The drawing under review shows one solid part. Ordinate dimensions are in mm from its lowest x, y, z. A direction names the side the tool comes from. Coordinates: 2 decimals unless noted, no trailing zeros. Write each loop counter-clockwise with the first axis right and the second up, starting at its lowest first coordinate (ties: lowest second). Pieces come first, ordered by that corner, then holes. Notation, with made-up numbers: (72, 13.25) - (93, 13.25) arc R20 ccw to (93, 50.25) - close; hole circle Ø2 at (61, -17.5). An arc over 180 degrees is marked (long way). Put each result on its own line as item: value. Start each with the question number.
Item 1: Consider section C-C on x = 86. Give the boundary of the cut face in (y, z), then the cut area to 3 significant figures.
Item 2: Consider section B-B on y = 80. Give the boundary of the cut face in (x, z).
Item 3: Machinability: for the marked faces 4, 5 and 6, which of the approach directions +Z, -Z, +X, -X, +Y, -Y give a long, thin tool a straight path to every point of the face, cutting with its end or side? Answer none if there is none.
Item 4: To check wall thickness, follow L1, parallel to Z at x = 8.5, y = 145; L2, parallel to Z at x = 92, y = 59. State the ranges of each line that lie inside material, in increasing order. Write a range as [from, to].
Item 5: Consider section A-A on x = 48.5. Give the boundary of the cut face in (y, z).
Item 6: Consider section D-D on y = 108.5. Give the boundary of the cut face in (x, z), then the cut area to 3 significant figures.
Item 7: For pin 1 (24 mm diameter, centred on x = 59.5, y = 77.5, fed in from -Z); pin 2 (16 mm diameter, centred on x = 77.5, z = 113, fed in from +Y); pin 3 (2.5 mm diameter, centred on x = 21, z = 12, fed in from +Y); pin 4 (24 mm diameter, centred on x = 94, y = 80, fed in from +Z), all flat-tipped, find the tip position at first contact; note any pin that passes through.
Item 8: Mouldability with a two-part tool opening along X and no side actions: class the marked faces 1, 2 and 3 as pulls with the +X half, pulls with the -X half, needs draft (parallel to the pull), parting line crosses it, or undercut.
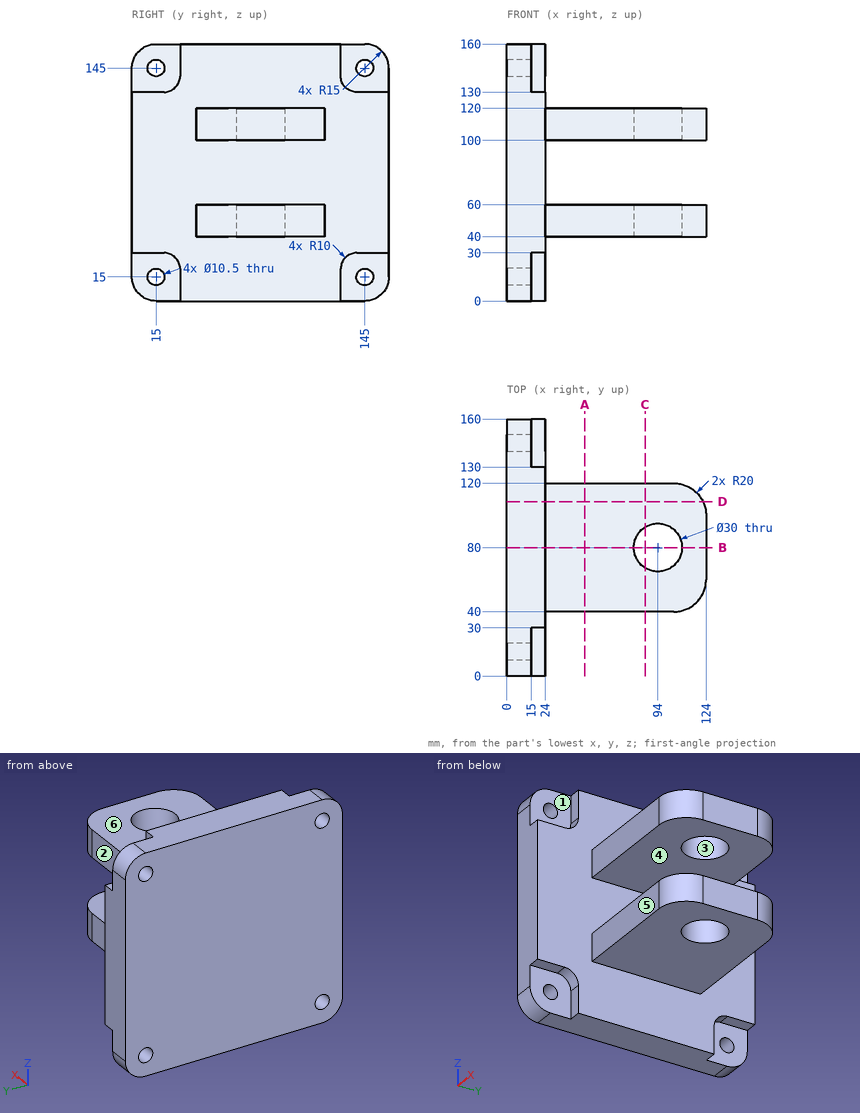
Report:
1. outline: (40, 40) - (67.31, 40) - (67.31, 60) - (40, 60) - close; (40, 100) - (67.31, 100) - (67.31, 120) - (40, 120) - close; (92.69, 40) - (120, 40) - (120, 60) - (92.69, 60) - close; (92.69, 100) - (120, 100) - (120, 120) - (92.69, 120) - close
1. area: 2,180 mm²
2. outline: (0, 0) - (24, 0) - (24, 40) - (79, 40) - (79, 60) - (24, 60) - (24, 100) - (79, 100) - (79, 120) - (24, 120) - (24, 160) - (0, 160) - close; (109, 40) - (124, 40) - (124, 60) - (109, 60) - close; (109, 100) - (124, 100) - (124, 120) - (109, 120) - close
3. face 4: +X, +Y, -Y
3. face 5: +Z, -Z, +X, -Y
3. face 6: +Z, +X, +Y, -Y
4. L1: [0, 9.75], [20.25, 139.75], [150.25, 160]
4. L2: [40, 60], [100, 120]
5. outline: (40, 40) - (120, 40) - (120, 60) - (40, 60) - close; (40, 100) - (120, 100) - (120, 120) - (40, 120) - close
6. outline: (0, 0) - (24, 0) - (24, 40) - (122.1, 40) - (122.1, 60) - (24, 60) - (24, 100) - (122.1, 100) - (122.1, 120) - (24, 120) - (24, 160) - (0, 160) - close
6. area: 7,760 mm²
7. pin 1: z = 40
7. pin 2: y = 120
7. pin 3: y = 130
7. pin 4: through
8. face 1: pulls with the +X half
8. face 2: needs draft
8. face 3: undercut
